Autodesk Inventor part; units mm, degrees
ref_plane "YZ Plane" through (0, 0, 0) normal (1, 0, 0) x (0, 1, 0)
ref_plane "XZ Plane" through (0, 0, 0) normal (0, 1, 0) x (-1, 0, 0)
ref_plane "XY Plane" through (0, 0, 0) normal (0, 0, 1) x (1, 0, 0)
sketch "Sketch1" plane through (0, 0, 0) normal (0, 0, 1) x (1, 0, 0)
  arc A0 (1.4424, 2.54) -> (1.4424, -2.54) centre (0, 0) ccw
  line L0 (1.4424, 2.54) -> (18.7855, 1.8463)
  line L1 (18.7855, -1.8463) -> (1.4424, -2.54)
  line L2 (20.4924, 0.0697) -> (20.4924, -0.0697)
  arc A1 (18.7855, -1.8463) -> (20.4924, -0.0697) centre (18.7144, -0.0697) ccw
  arc A2 (20.4924, 0.0697) -> (18.7855, 1.8463) centre (18.7144, 0.0697) ccw
  point P0 (20.4924, 1.778)
  point P1 (20.4924, -1.778)
  point P2 (20.4924, 0)
  dimension "d0" = 5.842
  dimension "d1" = 5.08
  dimension "d2" = 3.556
  dimension "d3" = 1.778
  dimension "d4" = 19.05
  dimension "d5" = 1.778
extrude "Extrusion1" add sketch "Sketch1" along normal blind 2.54
sketch "Sketch2" plane through (0, 0, 2.54) normal (0, 0, 1) x (1, 0, 0)
  circle A0 centre (0, 0) radius 2.921
extrude "Extrusion2" add sketch "Sketch2" along normal blind 1.016
sketch "Sketch3" plane through (0, 0, 3.556) normal (0, 0, 1) x (1, 0, 0)
  circle A0 centre (0, 0) radius 0.762
  circle A1 centre (0, 0) radius 1.524
  dimension "d10" = 1.524
  dimension "d11" = 0.762
extrude "Extrusion3" add sketch "Sketch3" along normal blind 12.7
sketch "Sketch4" plane through (0, 0, 3.556) normal (0, 0, 1) x (1, 0, 0)
  circle A0 centre (0, 0) radius 1.524
  line L0 (-1.0776, 1.0776) -> (-1.7252, 0.4301)
  line L1 (1.0776, -1.0776) -> (0.4301, -1.7252)
  arc A1 (-1.7252, 0.4301) -> (0.4301, -1.7252) centre (0, 0) ccw
  arc A2 (-1.0776, 1.0776) -> (1.0776, -1.0776) centre (0, 0) ccw
  dimension "d17" = 3.302
extrude "Extrusion5" add sketch "Sketch4" along normal blind 12.446 contours A0 L1 A1 L0
properties part number "Right leg distributor" material "Phenolic Resin"
CAD build for the part. Positions are in the model's coordinates, mm. A direction names the side the tool comes from. Round coordinates to 2 decimals unless told otherwise and drop trailing zeros. Order: outer loops, then holes, each group sorted by start corner. A loop starts at its lowest first (then second) coordinate and runs counter-clockwise, first axis right, second up. Notation, with made-up numbers: (84.5, -14) - (138.5, -14) arc R10 cw to (138.5, 1) - close; hole circle Ø5 at (20.25, 73). An arc over 180 degrees is marked (long way). Answer as CSV lines item,"result". Start each with the question number.
1. Saw through at A-A, the plane z = 13.25. Write the cut outline in (x, y), and give its area (3 significant figures).
2. Tool access for faces 4 (the face through (-2.92, -0.09, 1.25)), 5 (the face through (0, 0, 3.556)): list every direction of +Z, -Z, +X, -X, +Y, -Y with a clear straight run to the whole face (end or side of a thin tool).
3. Saw through at D-D, the plane x = 11.5. Write the cut outline in (y, z), and give its area (3 significant figures).
4. Saw through at C-C, the plane z = 2. Write the cut outline in (x, y), and give its area (3 significant figures).
5. Saw through at B-B, the plane x = 2.25. Write the cut outline in (y, z), and give its area (3 significant figures).
6. Pull direction X, two halves, no side cores. Call faces 1 (the face through (20, 1.3, 1.3)), 2 (the face through (-0.633, 2.852, 3.041)), 3 (the face through (-0.099, -0.756, 9.817)): +X half, -X half, draft (parallel to the pull), parting line (faces both ways), or undercut.
7. Drill centre lines: L1, parallel to Y at x = 0, z = 8; L2, parallel to Z at x = 19.25, y = -0.5; L3, parallel to Y at x = 0.5, z = 10.5. Where is each one in solid material? Low to high. Write a range as [from, to].
8. Pin check, flat tips, straight feed: pin 1 (1.5 mm diameter, centred on y = -0.5, z = 13.5, fed in from -X); pin 2 (8 mm diameter, centred on x = 13.5, z = 6.5, fed in from -Y); pin 3 (1.5 mm diameter, centred on x = 8, y = 0, fed in from +Z). Stop position of each tip, or through.
Model answer:
1,outline,"(-1.73, 0.43) arc R1.78 ccw to (0.43, -1.73) - (1.08, -1.08) arc R1.52 ccw to (-1.08, 1.08) - close; hole circle Ø1.52 at (0, 0)"
1,area,"6.48 mm²"
2,face 4,"+Z, -Z"
2,face 5,"+Z"
3,outline,"(-2.14, 0) - (2.14, 0) - (2.14, 2.54) - (-2.14, 2.54) - close"
3,area,"10.9 mm²"
4,outline,"(1.44, -2.54) - (18.79, -1.85) arc R1.78 ccw to (20.49, -0.07) - (20.49, 0.07) arc R1.78 ccw to (18.79, 1.85) - (1.44, 2.54) arc R2.92 ccw (long way) to start"
4,area,"102 mm²"
5,outline,"(-2.51, 0) - (2.51, 0) - (2.51, 2.54) - (1.86, 2.54) - (1.86, 3.56) - (-1.86, 3.56) - (-1.86, 2.54) - (-2.51, 2.54) - close"
5,area,"16.5 mm²"
6,face 1,"+X half"
6,face 2,"parting line"
6,face 3,"undercut"
7,L1,"y = [-1.78, -0.76], [0.76, 1.52]"
7,L2,"z = [0, 2.54]"
7,L3,"y = [-1.66, -0.58], [0.58, 1.44]"
8,pin 1,"stops at x = -1.78"
8,pin 2,"stops at y = -2.08"
8,pin 3,"stops at z = 2.54"
